```python
from build123d import *

# Parameters (mm, degrees)
F1_DEPTH  = 20
F2_W      = 20
F2_H      = 20
F3_DEPTH  = 20
F4_T      = -2.5
F5_R      = 2.5
F6_DEPTH  = 2.5
F7_R      = 2.5
F8_DEPTH  = 2.5
F9_R      = 2.5
F10_DEPTH = 2.5


with BuildPart() as f1:
    # F0 (on Front) → F1 (new body)
    with BuildSketch(Plane.XZ):
        Polygon((40, 0), (0, 0), (0, -40), (20, -40), (20, -20), (40, -20), align=None)
    extrude(amount=F1_DEPTH)

    # F2 (on face) → F3 (join)
    with BuildSketch(Plane.XZ.offset(20)):
        with Locations((10, -10)):
            Rectangle(F2_W, F2_H)
    extrude(amount=F3_DEPTH)

    # F4
    f4_openings = [f1.faces().sort_by_distance(p)[0] for p in [
        (10, -40, -10),
        (40, -10, -10),
        (10, -10, -40),
    ]]
    offset(amount=F4_T, openings=f4_openings, kind=Kind.INTERSECTION)

    # F5 (on face) → F6 (cut, through all)
    with BuildSketch(Plane(origin=(0, 0, 0), x_dir=(0, -1, 0), z_dir=(-1, 0, 0))):
        with Locations((30, -10)):
            Circle(F5_R)
        with Locations((10, -30)):
            Circle(F5_R)
    extrude(amount=-F6_DEPTH, mode=Mode.SUBTRACT)

    # F7 (on face) → F8 (cut, through all)
    with BuildSketch(Plane.XY):
        with Locations((10, -30)):
            Circle(F7_R)
        with Locations((30, -10)):
            Circle(F7_R)
    extrude(amount=-F8_DEPTH, mode=Mode.SUBTRACT)

    # F9 (on face) → F10 (cut, through all)
    with BuildSketch(Plane(origin=(0, 0, 0), x_dir=(-1, 0, 0), z_dir=(0, 1, 0))):
        with Locations((-30, -10)):
            Circle(F9_R)
        with Locations((-10, -30)):
            Circle(F9_R)
    extrude(amount=-F10_DEPTH, mode=Mode.SUBTRACT)


solid = f1.part
```
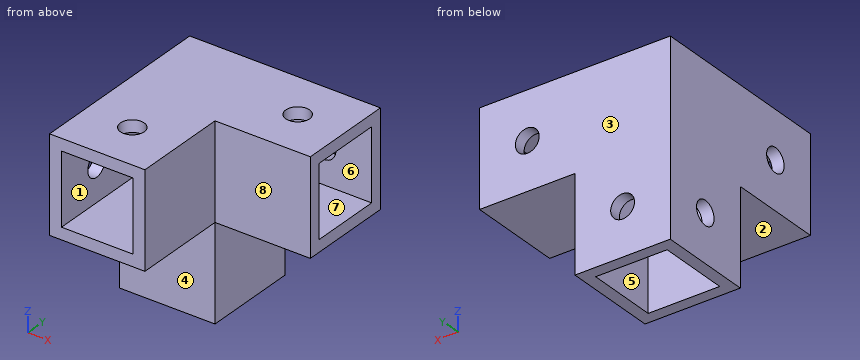
The model under review builds one solid part; all positions refer to its coordinate system, in mm. Face numbers are marked on the shaded views. A direction names the side the tool comes from. Coordinates: 2 decimals unless noted, no trailing zeros. Order: outer loops, then holes, each group sorted by start corner. A loop starts at its lowest first (then second) coordinate and runs counter-clockwise, first axis right, second up. Notation, with made-up numbers: (68.25, 73.5) -> (121.25, 73.5) arc R20 ccw to (121.25, 85.5) -> close; hole circle Ø4 at (74, -16.75). An arc over 180 degrees is marked (long way). Answer in a Markdown table with one row per item. Add a question column.
Item 1: Mouldability with a two-part tool opening along Z and no side actions: class the marked faces 1, 2 and 3 as +Z half, -Z half, draft (parallel to the pull), parting line (faces both ways), or undercut.
Item 2: We need section B-B on x = 10. Write out the cut boundary in (y, z).
Item 3: To check wall thickness, follow probe 1 along Z at (x, y) = (4.5, -22.5); probe 2 along X at (y, z) = (-34.5, -15.5); probe 3 along Z at (x, y) = (30, -1). State the ranges of each line that lie inside material, in increasing order.
Item 4: Machinability: for the marked faces 4, 5, 6, 7 and 8, which of the approach directions +Z, -Z, +X, -X, +Y, -Y give a long, thin tool a straight path to every point of the face, cutting with its end or side? Answer none if there is none.
Item 5: We need section C-C on y = -14. Write out the cut boundary in (x, z).
Item 6: We need section A-A on z = -10. Write out the cut boundary in (x, y).
Item 7: Clearance check with flat-ended pins moving along their axes: pin 1 (3 mm diameter, centred on x = 14, y = -26.5, fed in from -Z); pin 2 (6 mm diameter, centred on y = -10, z = -30, fed in from +X); pin 3 (4.5 mm diameter, centred on x = 10, z = -30, fed in from +Y); pin 4 (10 mm diameter, centred on y = -29, z = -28.5, fed in from -X). State where each tip first meets the part, or that it passes through.
Final values:
| question | item | result |
|---|---|---|
| 1 | face 1 | undercut |
| 1 | face 2 | -Z half |
| 1 | face 3 | draft |
| 2 | outline | (-40, -20) -> (-20, -20) -> (-20, -40) -> (-17.5, -40) -> (-17.5, -17.5) -> (-40, -17.5) -> close; (-40, -2.5) -> (-32.5, -2.5) -> (-32.5, 0) -> (-40, 0) -> close; (-27.5, -2.5) -> (-2.5, -2.5) -> (-2.5, -27.5) -> (0, -27.5) -> (0, 0) -> (-27.5, 0) -> close; (-2.5, -40) -> (0, -40) -> (0, -32.5) -> (-2.5, -32.5) -> close |
| 3 | probe 1 | z = -20 to -17.5, -2.5 to 0 |
| 3 | probe 2 | x = 0 to 2.5, 17.5 to 20 |
| 3 | probe 3 | z = -20 to -12.5, -7.5 to 0 |
| 4 | face 4 | -Z, +X, -X, -Y |
| 4 | face 5 | -Z |
| 4 | face 6 | none |
| 4 | face 7 | +X |
| 4 | face 8 | +Z, -Z, +X, -Y |
| 5 | outline | (0, -40) -> (2.5, -40) -> (2.5, -2.5) -> (40, -2.5) -> (40, 0) -> (0, 0) -> close; (17.5, -40) -> (20, -40) -> (20, -20) -> (40, -20) -> (40, -17.5) -> (17.5, -17.5) -> close |
| 6 | outline | (0, -40) -> (2.5, -40) -> (2.5, -32.5) -> (0, -32.5) -> close; (0, -27.5) -> (2.5, -27.5) -> (2.5, -2.5) -> (27.5, -2.5) -> (27.5, 0) -> (0, 0) -> close; (17.5, -40) -> (20, -40) -> (20, -20) -> (40, -20) -> (40, -17.5) -> (17.5, -17.5) -> close; (32.5, -2.5) -> (40, -2.5) -> (40, 0) -> (32.5, 0) -> close |
| 7 | pin 1 | stops at z = -20 |
| 7 | pin 2 | stops at x = 20 |
| 7 | pin 3 | stops at y = -17.5 |
| 7 | pin 4 | passes through |
